The model under review builds one solid part; all positions refer to its coordinate system, in mm. Face numbers are marked on the shaded views. A direction names the side the tool comes from. Give positions to 0.01 mm unless a question says otherwise; leave off trailing zeros. Loops run counter-clockwise (first coordinate to the right, second up) from the corner with the lowest first, then second, coordinate; pieces in that order, holes last. Notation, with made-up numbers: (-10, -1) - (2, -1) arc R36 ccw to (2, 38) - close; hole circle Ø1 at (-30, -26.5). An arc over 180 degrees is marked (long way). Return JSON: item names as keys, results as strings. Group by question number.
```python
from build123d import *

# Parameters (mm, degrees)
SKETCH3_W           = 160
SKETCH3_H           = 12
BOSS_EXTRUDE2_DEPTH = 26
SKETCH4_W           = 160
SKETCH4_H           = 12
BOSS_EXTRUDE3_DEPTH = 12
SKETCH5_W           = 160
SKETCH5_H           = 12
BOSS_EXTRUDE4_DEPTH = 12
SKETCH8_R           = 15
BOSS_EXTRUDE5_DEPTH = 52
RIB1_REACH          = 120.017
SKETCH14_WALL_W     = 346.495870774
SKETCH14_WALL_H     = 12


with BuildPart() as part:
    # Sketch3 → Boss-Extrude2 (new, symmetric)
    with BuildSketch(Plane.XY):
        Rectangle(SKETCH3_W, SKETCH3_H)
    extrude(amount=BOSS_EXTRUDE2_DEPTH, both=True)

    # Sketch4 → Boss-Extrude3 (add, symmetric)
    with BuildSketch(Plane.XY.offset(26)):
        with Locations((0, -12)):
            Rectangle(SKETCH4_W, SKETCH4_H)
    extrude(amount=BOSS_EXTRUDE3_DEPTH, both=True)

    # Sketch5 → Boss-Extrude4 (add, symmetric)
    with BuildSketch(Plane(origin=(0, 0, -26), x_dir=(-1, 0, 0), z_dir=(0, 0, -1))):
        with Locations((0, -12)):
            Rectangle(SKETCH5_W, SKETCH5_H)
    extrude(amount=BOSS_EXTRUDE4_DEPTH, both=True)

    # Sketch8 → Boss-Extrude5 (add)
    with BuildSketch(Plane(origin=(0, 0, -26), x_dir=(-1, 0, 0), z_dir=(0, 0, -1))):
        with BuildLine():
            Line((20, 6), (80, 6))
            Line((80, 6), (80, 48))
            ThreePointArc((80, 48), (50, 78), (20, 48))
            Line((20, 48), (20, 6))
        make_face()
        with Locations((50, 48)):
            Circle(SKETCH8_R, mode=Mode.SUBTRACT)
    extrude(amount=-BOSS_EXTRUDE5_DEPTH)

    # Sketch14 wall → Rib1 (add, up to next)
    with BuildSketch(Plane(origin=(30, 27, 0), x_dir=(0.921982105607, -0.387232484355, 0), z_dir=(0.387232484355, 0.921982105607, 0)), mode=Mode.PRIVATE) as rib1_sk1:
        Rectangle(SKETCH14_WALL_W, SKETCH14_WALL_H)
    rib1_tool1 = extrude(rib1_sk1.sketch, amount=-RIB1_REACH, mode=Mode.PRIVATE) - part.part
    add(rib1_tool1.solids().sort_by_distance((30, 27, 0))[0])


solid = part.part
```
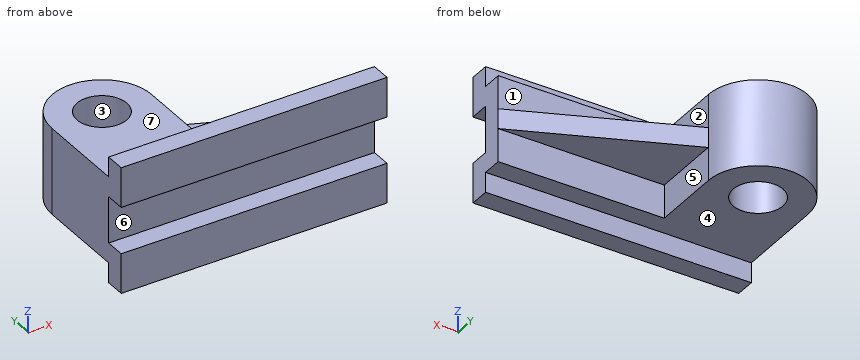
1) We need section C-C, the plane y = 35.5. Write out the cut boundary in (x, z), plus the area to 3 significant figures.
2) We need section B-B, the plane x = -50. Write out the cut boundary in (y, z).
3) We need section A-A, the plane z = 19. Write out the cut boundary in (x, y), plus the area to 3 significant figures.
4) For pin 1 Ø3 at (x, z) = (34.5, -4.5) entering from -Y; pin 2 Ø1 at (y, z) = (36.5, -18) entering from +X; pin 3 Ø3.5 at (x, z) = (20, -30) entering from +Y; pin 4 Ø6 at (x, y) = (35.5, 31) entering from +Z, all flat-tipped, find the tip position at first contact; note any pin that passes through.
5) We need section D-D, the plane x = 61. Write out the cut boundary in (y, z).
6) Draft analysis for pull direction X (two halves, no side actions). For the marked faces 1, 2 and 3, state which applies: +X half, -X half, draft (parallel to the pull), parting line (faces both ways), or undercut.
7) Tool access review of the marked faces 4, 5, 6 and 7: name each direction out of +Z, -Z, +X, -X, +Y, -Y from which nothing blocks a thin tool from reaching the whole face with its end or side.
8) To check wall thickness, follow line 1 (Y direction, x = -50, z = 15); line 2 (Y direction, x = -50, z = -8.5); line 3 (Z direction, x = 10, y = -12.5). State the ranges of each line that lie inside material, in increasing order.
Findings:
{
 "1": {"outline": "(-80, -26) - (-58.29, -26) - (-58.29, 26) - (-80, 26) - close; (-41.71, -26) - (-20, -26) - (-20, -6) - (9.76, -6) - (9.76, 6) - (-20, 6) - (-20, 26) - (-41.71, 26) - close", "area": "2,610 mm^2"},
 "2": {"outline": "(-18, -38) - (-6, -38) - (-6, -26) - (33, -26) - (33, 26) - (-6, 26) - (-6, 38) - (-18, 38) - (-18, 14) - (-6, 14) - (-6, -14) - (-18, -14) - close; (63, -26) - (78, -26) - (78, 26) - (63, 26) - close"},
 "3": {"outline": "(-80, -18) - (80, -18) - (80, 6) - (-20, 6) - (-20, 48) arc R30 ccw to (-80, 48) - close; hole circle Ø30 at (-50, 48)", "area": "7,070 mm^2"},
 "4": {"pin 1": "stops at y = -6", "pin 2": "stops at x = -20", "pin 3": "stops at y = -6", "pin 4": "passes through"},
 "5": {"outline": "(-18, -38) - (-6, -38) - (-6, -26) - (6, -26) - (6, -6) - (13.98, -6) - (13.98, 6) - (6, 6) - (6, 26) - (-6, 26) - (-6, 38) - (-18, 38) - (-18, 14) - (-6, 14) - (-6, -14) - (-18, -14) - close"},
 "6": {"face 1": "draft", "face 2": "+X half", "face 3": "undercut"},
 "7": {"face 4": "-Z, +X, -X, +Y", "face 5": "-Z, +X, +Y", "face 6": "+X, -X, -Y", "face 7": "+Z, +X, -X, +Y"},
 "8": {"line 1": "y = -18 to 33, 63 to 78", "line 2": "y = -6 to 33, 63 to 78", "line 3": "z = -38 to -14, 14 to 38"}
}
